Here's how the part is built. I have some questions about the finished solid (model axes, mm). Round coordinates to 2 decimals unless told otherwise and drop trailing zeros. Write each loop counter-clockwise with the first axis right and the second up, starting at its lowest first coordinate (ties: lowest second). Pieces come first, ordered by that corner, then holes. Notation, with made-up numbers: (34.5, 18.5) -> (51.5, 18.5) arc R19 ccw to (51.5, 25.5) -> close; hole circle Ø3 at (13, 23). An arc over 180 degrees is marked (long way). Answer in a Markdown table with one row per item.
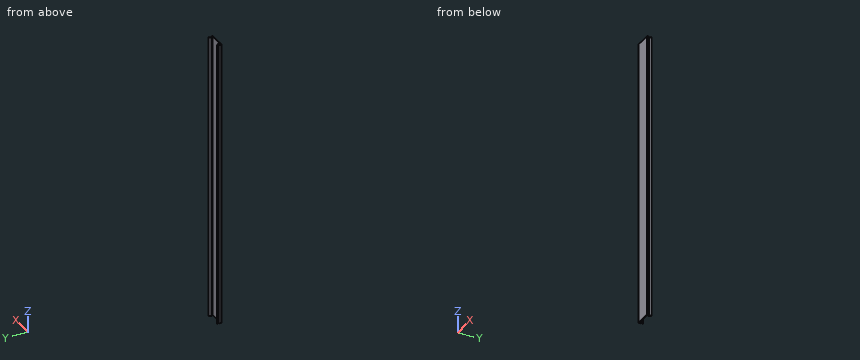
from build123d import *

# Parameters (mm, degrees)
BOSS_EXTRUDE1_DEPTH = 360


with BuildPart() as part:
    # Sketch1 → Boss-Extrude1 (new, symmetric)
    with BuildSketch(Plane.XY):
        with BuildLine():
            Line((46.962560252, -71.288832462), (46.962560252, -67.53553159))
            ThreePointArc((46.962560252, -67.53553159), (46.588231361, -66.507071414), (45.640397337, -65.959839185))
            Line((45.640397337, -65.959839185), (43.510465799, -65.584274788))
            ThreePointArc((43.510465799, -65.584274788), (43.278063156, -65.384023859), (43.343154142, -65.084232954))
            Line((43.343154142, -65.084232954), (46.795419695, -61.382131396))
            ThreePointArc((46.795419695, -61.382131396), (46.763338723, -60.463452556), (45.844659883, -60.495533528))
            Line((45.844659883, -60.495533528), (42.231206551, -64.370487816))
            ThreePointArc((42.231206551, -64.370487816), (42.032142684, -64.68598495), (41.962560252, -65.052486177))
            Line((41.962560252, -65.052486177), (41.962560252, -65.288832462))
            ThreePointArc((41.962560252, -65.288832462), (42.336889143, -66.317292637), (43.284723168, -66.864524867))
            Line((43.284723168, -66.864524867), (45.414654706, -67.240089264))
            ThreePointArc((45.414654706, -67.240089264), (45.592373585, -67.342695307), (45.662560252, -67.53553159))
            Line((45.662560252, -67.53553159), (45.662560252, -69.988832462))
            Line((45.662560252, -69.988832462), (8.262560252, -69.988832462))
            Line((8.262560252, -69.988832462), (8.262560252, -67.53553159))
            ThreePointArc((8.262560252, -67.53553159), (8.332746919, -67.342695307), (8.510465799, -67.240089264))
            Line((8.510465799, -67.240089264), (10.640397337, -66.864524867))
            ThreePointArc((10.640397337, -66.864524867), (11.588231361, -66.317292637), (11.962560252, -65.288832462))
            Line((11.962560252, -65.288832462), (11.962560252, -65.052486177))
            ThreePointArc((11.962560252, -65.052486177), (11.89297782, -64.68598495), (11.693913954, -64.370487816))
            Line((11.693913954, -64.370487816), (8.080460622, -60.495533528))
            ThreePointArc((8.080460622, -60.495533528), (7.161781782, -60.463452556), (7.12970081, -61.382131396))
            Line((7.12970081, -61.382131396), (10.581966363, -65.084232954))
            ThreePointArc((10.581966363, -65.084232954), (10.647057349, -65.384023859), (10.414654706, -65.584274788))
            Line((10.414654706, -65.584274788), (8.284723168, -65.959839185))
            ThreePointArc((8.284723168, -65.959839185), (7.336889143, -66.507071414), (6.962560252, -67.53553159))
            Line((6.962560252, -67.53553159), (6.962560252, -71.288832462))
            Line((6.962560252, -71.288832462), (46.962560252, -71.288832462))
        make_face()
    extrude(amount=BOSS_EXTRUDE1_DEPTH, both=True)


solid = part.part
1) I want a section at B-B, the plane x = 21. List the corners of the cut face in (y, z) for me, and give its area (3 significant figures).
Response:
| item | result |
|---|---|
| outline | (-71.29, -360) -> (-69.99, -360) -> (-69.99, 360) -> (-71.29, 360) -> close |
| area | 936 mm^2 |
2) I want a section at A-A, the plane z = -52.5. List the corners of the cut face in (x, y) for me, and give its area (3 significant figures).
Response:
| item | result |
|---|---|
| outline | (6.96, -71.29) -> (46.96, -71.29) -> (46.96, -67.54) arc R1.6 ccw to (45.64, -65.96) -> (43.51, -65.58) arc R0.3 cw to (43.34, -65.08) -> (46.8, -61.38) arc R0.65 ccw to (45.84, -60.5) -> (42.23, -64.37) arc R1 ccw to (41.96, -65.05) -> (41.96, -65.29) arc R1.6 ccw to (43.28, -66.86) -> (45.41, -67.24) arc R0.3 cw to (45.66, -67.54) -> (45.66, -69.99) -> (8.26, -69.99) -> (8.26, -67.54) arc R0.3 cw to (8.51, -67.24) -> (10.64, -66.86) arc R1.6 ccw to (11.96, -65.29) -> (11.96, -65.05) arc R1 ccw to (11.69, -64.37) -> (8.08, -60.5) arc R0.65 ccw to (7.13, -61.38) -> (10.58, -65.08) arc R0.3 cw to (10.41, -65.58) -> (8.28, -65.96) arc R1.6 ccw to (6.96, -67.54) -> close |
| area | 87.3 mm^2 |
3) I need wall thicknesses on line 1 (X direction, y = -65, z = -324); line 2 (X direction, y = -67.5, z = -67); line 3 (Y direction, x = 10.5, z = 50). Which ranges of each line are inside material? Lowest first, please. Write a range as [from, to].
Response:
| item | result |
|---|---|
| line 1 | x = [10.5, 11.96], [41.96, 43.42] |
| line 2 | x = [6.96, 8.26], [45.66, 46.96] |
| line 3 | y = [-71.29, -69.99], [-66.89, -65.56], [-65, -63.09] |
4) For pin 1 (2 mm diameter, centred on y = -68.5, z = -85, fed in from +X); pin 2 (1.5 mm diameter, centred on x = 18.5, z = 193, fed in from +Y); pin 3 (18.5 mm diameter, centred on x = 33.5, z = 35, fed in from +Y), each with a flat end and sliding along its axis, tell me the tip position at first contact or that it passes through.
Response:
| item | result |
|---|---|
| pin 1 | stops at x = 46.96 |
| pin 2 | stops at y = -69.99 |
| pin 3 | stops at y = -63.81 |
